Autodesk Fusion 360 part; units mm, degrees
sketch "Sketch1" plane through (0, 0, 0) normal (0, 1, 0) x (1, 0, 0)
  circle A0 centre (0, 0) radius 15
  dimension "d1" = 30
extrude "Extrude1" add sketch "Sketch1" along normal blind 3.5
ref_plane "WorkPlane1" through (0, 3.5, 0) normal (0, 1, 0) x (1, 0, 0)
sketch "Sketch2" plane through (0, 3.5, 0) normal (0, 1, 0) x (1, 0, 0)
  circle A0 centre (0, 0) radius 9.2075
  dimension "d5" = 18.415
extrude "Extrude2" add sketch "Sketch2" along normal blind 7
ref_plane "WorkPlane2" through (0, 3.5, 0) normal (0, 1, 0) x (1, 0, 0)
sketch "Sketch3" plane through (0, 3.5, 0) normal (0, 1, 0) x (1, 0, 0)
  circle A0 centre (0, 0) radius 15
  circle A1 centre (0, 0) radius 13.2
  dimension "d9" = 26.4
extrude "Extrude3" add sketch "Sketch3" along normal blind 14
Design review of the part built by this model. Coordinates are the model's own, in mm. A direction names the side the tool comes from. Give positions to 0.01 mm unless a question says otherwise; leave off trailing zeros. Order: outer loops, then holes, each group sorted by start corner. A loop starts at its lowest first (then second) coordinate and runs counter-clockwise, first axis right, second up. Notation, with made-up numbers: M -8,40 L 37,40 A19 ccw 37,76 Z; hole C 7,33 d1. An arc over 180 degrees is marked long. One line per question, with ' | ' between items. Start each with the question number.
Q1. The part is to be moulded in two halves that separate along X. For faces 3 (the face through (3, 3.5, -9)), 4 (the face through (-14.985, 8.628, 0.66)), 5 (the face through (9, 17.5, 10)), 6 (the face through (-7.31, 6.95, -5.6)), say which applies: +X half, -X half, draft (parallel to the pull), parting line (faces both ways), or undercut.
Q2. We need section C-C (z = 0). Write out the cut boundary in (x, y).
Q3. For L1, parallel to X at y = 7.25, z = 0; L2, parallel to Z at x = 0, y = 10.75, list the stretches that pass through material, from the lowest coordinate up. Write a range as [from, to].
Q4. We need section B-B (y = 4.25). Write out the cut boundary in (x, z) (1 decimal), plus the area to 3 significant figures.
Q5. For pin 1 Ø3 at (x, y) = (-11.5, 13.5) entering from -Z; pin 2 Ø4 at (y, z) = (7.5, -9) entering from +X; pin 3 Ø4 at (y, z) = (15, -8) entering from +X, all flat-tipped, find the tip position at first contact; note any pin that passes through.
Q6. We need section A-A (x = 0). Write out the cut boundary in (y, z).
Q7. We need section D-D (y = 12.5). Write out the cut boundary in (x, z).
Q8. Machinability: for faces 1 (the face through (0, 10.5, 0)), 2 (the face through (0, 0, 0)), which of the approach directions +Z, -Z, +X, -X, +Y, -Y give a long, thin tool a straight path to every point of the face, cutting with its end or side? Answer none if there is none.
Returned:
1) face 3: undercut | face 4: parting line | face 5: draft | face 6: undercut
2) outline: M -15,0 L 15,0 L 15,17.5 L 13.2,17.5 L 13.2,3.5 L 9.21,3.5 L 9.21,10.5 L -9.21,10.5 L -9.21,3.5 L -13.2,3.5 L -13.2,17.5 L -15,17.5 Z
3) L1: [-15, -13.2], [-9.21, 9.21], [13.2, 15] | L2: [-15, -13.2], [13.2, 15]
4) outline: C 0,0 d30; C 0,0 d18.4; hole C 0,0 d26.4 | area: 426 mm2
5) pin 1: z = -11.18 | pin 2: x = 13.27 | pin 3: x = 13.75
6) outline: M 0,-15 L 17.5,-15 L 17.5,-13.2 L 3.5,-13.2 L 3.5,-9.21 L 10.5,-9.21 L 10.5,9.21 L 3.5,9.21 L 3.5,13.2 L 17.5,13.2 L 17.5,15 L 0,15 Z
7) outline: C 0,0 d30; hole C 0,0 d26.4
8) face 1: +Y | face 2: +Z, -Z, +X, -X, -Y
